Geometry check sheet. Reference: the model listing, model coordinates, mm. Coordinates: 2 decimals unless noted, no trailing zeros. Order: outer loops, then holes, each group sorted by start corner. A loop starts at its lowest first (then second) coordinate and runs counter-clockwise, first axis right, second up. Notation, with made-up numbers: (57.25, 66) - (114.25, 66) arc R28 ccw to (114.25, 92) - close; hole circle Ø5 at (-0.75, 36.5). An arc over 180 degrees is marked (long way). Put each result on its own line as item: value.
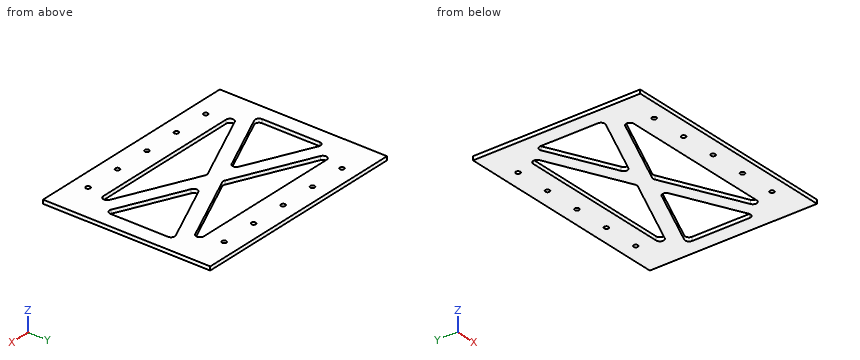
Autodesk Inventor part; units mm, degrees
ref_plane "YZ Plane" through (0, 0, 0) normal (1, 0, 0) x (0, 1, 0)
ref_plane "XZ Plane" through (0, 0, 0) normal (0, 1, 0) x (-1, 0, 0)
ref_plane "XY Plane" through (0, 0, 0) normal (0, 0, 1) x (1, 0, 0)
sketch "profile sketch" plane through (0, 0, 0) normal (0, 0, 1) x (1, 0, 0)
  line L0 (0, 0) -> (180.34, 0)
  line L1 (180.34, 0) -> (180.34, 136.5504)
  line L2 (180.34, 136.5504) -> (0, 136.5504)
  line L3 (0, 136.5504) -> (0, 0)
  dimension "d5" = 180.34
  dimension "d6" = 136.5504
extrude "Plate1" add sketch "profile sketch" along normal blind 3.048
sketch "rv_hole_sketch" plane through (0, 0, 3.048) normal (0, 0, 1) x (1, 0, 0)
  line L0 (0, 136.5504) -> (0, 0) construction
  line L1 (180.34, 0) -> (180.34, 136.5504) construction
  line L2 (0, 136.5504) -> (180.34, 136.5504) construction
  line L3 (180.34, 0) -> (0, 0) construction
  line L4 (0, 123.8504) -> (30.0567, 123.8504) construction
  line L5 (30.0567, 123.8504) -> (60.1133, 123.8504) construction
  line L6 (60.1133, 123.8504) -> (90.17, 123.8504) construction
  line L7 (90.17, 123.8504) -> (120.2267, 123.8504) construction
  line L8 (120.2267, 123.8504) -> (150.2833, 123.8504) construction
  line L9 (150.2833, 123.8504) -> (180.34, 123.8504) construction
  line L10 (0, 12.7) -> (30.0567, 12.7) construction
  line L11 (30.0567, 12.7) -> (60.1133, 12.7) construction
  line L12 (60.1133, 12.7) -> (90.17, 12.7) construction
  line L13 (90.17, 12.7) -> (120.2267, 12.7) construction
  line L14 (120.2267, 12.7) -> (150.2833, 12.7) construction
  line L15 (150.2833, 12.7) -> (180.34, 12.7) construction
  dimension "d10" = 12.7
  dimension "d11" = 12.7
hole "rv_holes" at (30.0567, 123.8504, 3.048) at (60.1133, 123.8504, 3.048) at (90.17, 123.8504, 3.048) at (120.2267, 123.8504, 3.048) at (150.2833, 123.8504, 3.048) at (150.2833, 12.7, 3.048) at (120.2267, 12.7, 3.048) at (90.17, 12.7, 3.048) at (60.1133, 12.7, 3.048) at (30.0567, 12.7, 3.048) direction (0, 0, -1) diameter 3.5719 depth 3.048 tip angle 118
sketch "cutout_sketch" plane through (0, 0, 3.048) normal (0, 0, 1) x (1, 0, 0)
  line L0 (12.7, 109.3645) -> (90.17, 74.6252)
  line L1 (90.17, 74.6252) -> (167.64, 109.3645)
  line L2 (167.64, 109.3645) -> (12.7, 109.3645)
  line L3 (12.7, 27.1859) -> (90.17, 61.9252)
  line L4 (90.17, 61.9252) -> (167.64, 27.1859)
  line L5 (167.64, 27.1859) -> (12.7, 27.1859)
  circle A0 centre (90.17, 123.8504) radius 1.7859
  circle A1 centre (90.17, 12.7) radius 1.7859
  line L6 (0, 0) -> (0, 136.5504)
  line L7 (180.34, 136.5504) -> (180.34, 0)
  line L8 (90.17, 74.6252) -> (90.17, 61.9252) construction
  line L9 (12.7, 96.6645) -> (76.0092, 68.2752)
  line L10 (76.0092, 68.2752) -> (12.7, 39.8859)
  line L11 (12.7, 39.8859) -> (12.7, 96.6645)
  line L12 (167.64, 96.6645) -> (104.3308, 68.2752)
  line L13 (104.3308, 68.2752) -> (167.64, 39.8859)
  line L14 (167.64, 39.8859) -> (167.64, 96.6645)
  line L15 (167.64, 109.3645) -> (167.64, 27.1859) construction
  line L16 (12.7, 109.3645) -> (12.7, 27.1859) construction
  dimension "d36" = 12.7
  dimension "d37" = 12.7
  dimension "d38" = 12.7
  dimension "d39" = 12.7
  dimension "d40" = 12.7
  dimension "d41" = 12.7
  dimension "d42" = 12.7
  dimension "d43" = 12.7
extrude "Cut2" cut sketch "cutout_sketch" against normal blind 3.048 contours L2 L1 L0 | L3 L4 L5 | L9 L10 L11 | L14 L13 L12
fillet "Corner Round3" radius 3.175 12 edges at (12.7, 109.3645, 1.524) (167.64, 109.3645, 1.524) (90.17, 74.6252, 1.524) (12.7, 39.8859, 1.524) (12.7, 96.6645, 1.524) (76.0092, 68.2752, 1.524) (90.17, 61.9252, 1.524) (12.7, 27.1859, 1.524) (167.64, 27.1859, 1.524) (104.3308, 68.2752, 1.524) (167.64, 96.6645, 1.524) (167.64, 39.8859, 1.524)
equation "\"d5\" = bh_length"
equation "\"d6\" = bp_height"
equation "\"d10\" = 0.5 * cb_outer_diameter"
equation "\"d11\" = 0.5 * cb_outer_diameter"
equation "\"d12\" = rv_hole_diameter"
equation "\"d17\" = Thickness"
equation "\"d36\" = cmp_mounting_margins"
equation "\"d37\" = cmp_mounting_margins"
equation "\"d38\" = cmp_mounting_margins"
equation "\"d39\" = cmp_mounting_margins"
equation "\"d40\" = cmp_mounting_margins"
equation "\"d41\" = cmp_mounting_margins"
equation "\"d42\" = cmp_mounting_margins"
equation "\"d43\" = cmp_mounting_margins"
equation "\"d44\" = Thickness"
equation "\"d46\" = spd_fillet_size"
equation "\"BendRadius\" = Thickness"
equation "\"BendReliefWidth\" = Thickness"
equation "\"BendReliefDepth\" = 0.5 * Thickness"
equation "\"CornerReliefSize\" = 4 * Thickness"
equation "\"MinimumRemnant\" = 2 * Thickness"
equation "\"TransitionRadius\" = BendRadius"
equation "\"JacobiRadiusSize\" = BendRadius"
equation "\"GapSize\" = Thickness"
equation "\"bh_width\" = 87.63"
equation "\"bh_length\" = 180.34"
equation "\"bh_height\" = bp_height - cb_outer_diameter"
equation "\"bh_metal_width\" = 1.5875"
equation "\"cpn_diameter\" = 69.85"
equation "\"cpn_length\" = 311.15"
equation "\"cmp_foot_seperation_long\" = 139.954"
equation "\"cmp_foot_seperation_short\" = 36.068"
equation "\"cmp_mounting_margins\" = 12.7"
equation "\"cmp_foot_bolt_diameter\" = 6.35"
equation "\"spd_fillet_size\" = 3.175"
equation "\"bp_height\" = gb_mh_seperation + st_outer_diameter"
equation "\"bp_tensioner_width\" = 6.35"
equation "\"bp_tensioner_height\" = 50.8"
equation "\"bp_tensioner_wood_mount_from_tensioner_top\" = 12.7"
equation "\"bp_tensioner_wood_mount_diameter\" = 6.35"
equation "\"cb_outer_diameter\" = 25.4"
equation "\"cb_wall_thickness\" = 1.5875"
equation "\"cb_length\" = 457.2"
equation "\"pdb_mounting_holes_short\" = 104.394"
equation "\"cb_pdb_low_mount_offset\" = 16.0782"
equation "\"pdb_mounting_holes_long\" = 182.2704"
equation "\"pdb_ziptie_hole_diameter\" = 6.35"
equation "\"gb_mh_seperation\" = 111.1504"
equation "\"gb_mh_diameter\" = 6.35"
equation "\"gb_axle_from_edge\" = 38.1"
equation "\"gb_width\" = 127"
equation "\"gb_bearing_diameter\" = 28.575"
equation "\"gb_to_bottom_of_side_assembly\" = 4.7752"
equation "\"ncbt_rivet_row_length\" = 114.3"
equation "\"rv_hole_diameter\" = 3.57187"
equation "\"st_outer_diameter\" = 25.4"
equation "\"st_wall_thickness\" = 1.5875"
equation "\"st_length\" = 685.8"
equation "\"st_gbmh_from_center\" = 55.5752"
equation "\"st_cutout_depth_right\" = 203.2"
equation "\"st_cutout_depth_left\" = 203.2"
equation "\"st_rivet_distance\" = 19.05"
equation "\"so_inner_diameter\" = 7.62"
equation "\"so_wall_thickness\" = 5.08"
equation "\"so_length\" = 40.64"
equation "\"twb_width\" = st_outer_diameter"
equation "\"twb_length\" = bp_tensioner_width + 2 * twb_margin_on_each_side"
equation "\"twb_height\" = 2 * bp_tensioner_wood_mount_diameter + bp_tensioner_height + 2 * bp_tensioner_wood_mount_from_tensioner_top + twb_margin_on_each_side"
equation "\"twb_margin_on_each_side\" = 6.35"
equation "\"twb_tensioner_from_edge\" = -0.5 * bp_tensioner_height + 0.5 * twb_height"
equation "\"tb_rivet_row_length\" = 127"
equation "\"bp_thickness\" = 3.048"
equation "\"bp_width\" = 76.2"
equation "\"bp_axle_height\" = 45.1612"
equation "\"magic_axle_offset\" = 2.286"
equation "\"bp_tensioner_from_bottom\" = 38.1"
equation "\"bp_tensioner_from_side\" = 25.4"
equation "\"d7\" = BendRadius"
equation "\"bh_alternate_height\" = 25.4"
equation "\"bh_alternate_width\" = 81.28"
equation "\"tb_metal_thickness\" = 3.048"
equation "\"tb_hm_mounting_slot_length\" = 40.64"
equation "\"gb_mh_seperation_alt\" = 111.125"
equation "\"gb_axle_from_edge_alt\" = 43.1546"
equation "\"bp_axle_height_alt\" = 50.2158"
equation "\"pdb_mount_include\" = 0"
properties part number "cross_structural_plate(csp)" material "Aluminum 6061"
Q1. Thickness scan on L1, parallel to X at y = 12.7, z = 1.9; L2, parallel to Y at x = 90.17, z = 1.4; L3, parallel to Y at x = 82.5, z = 2.75. Record the ranges inside material, lowest first. Write a range as [from, to].
Answer block:
L1: x = [0, 28.27], [31.84, 58.33], [61.9, 88.38], [91.96, 118.44], [122.01, 148.5], [152.07, 180.34]
L2: y = [0, 10.91], [14.49, 27.19], [61.62, 74.93], [109.36, 122.06], [125.64, 136.55]
L3: y = [0, 27.19], [58.49, 78.06], [109.36, 136.55]
Q2. Section check C-C on y = 68.5. Record the boundary of the cut face in (x, z).
Answer block:
outline: (0, 0) - (12.7, 0) - (12.7, 3.05) - (0, 3.05) - close; (71.42, 0) - (108.92, 0) - (108.92, 3.05) - (71.42, 3.05) - close; (167.64, 0) - (180.34, 0) - (180.34, 3.05) - (167.64, 3.05) - close
Q3. Section check D-D on x = 102. Record the boundary of the cut face in (y, z), then the cut area to 3 significant figures.
Answer block:
outline: (0, 0) - (27.19, 0) - (27.19, 3.05) - (0, 3.05) - close; (56.62, 0) - (79.93, 0) - (79.93, 3.05) - (56.62, 3.05) - close; (109.36, 0) - (136.55, 0) - (136.55, 3.05) - (109.36, 3.05) - close
area: 237 mm^2
Q4. Section check B-B on y = 47.5. Record the boundary of the cut face in (x, z), then the cut area to 3 significant figures.
Answer block:
outline: (0, 0) - (12.7, 0) - (12.7, 3.05) - (0, 3.05) - close; (29.68, 0) - (58, 0) - (58, 3.05) - (29.68, 3.05) - close; (122.34, 0) - (150.66, 0) - (150.66, 3.05) - (122.34, 3.05) - close; (167.64, 0) - (180.34, 0) - (180.34, 3.05) - (167.64, 3.05) - close
area: 250 mm^2
Q5. Section check A-A on x = 135. Record the boundary of the cut face in (y, z), then the cut area to 3 significant figures.
Answer block:
outline: (0, 0) - (27.19, 0) - (27.19, 3.05) - (0, 3.05) - close; (41.82, 0) - (54.52, 0) - (54.52, 3.05) - (41.82, 3.05) - close; (82.03, 0) - (94.73, 0) - (94.73, 3.05) - (82.03, 3.05) - close; (109.36, 0) - (136.55, 0) - (136.55, 3.05) - (109.36, 3.05) - close
area: 243 mm^2
